Build history of the part. All positions in model axes, mm. A direction names the side the tool comes from. Give positions to 0.01 mm unless a question says otherwise; leave off trailing zeros. Write each loop counter-clockwise with the first axis right and the second up, starting at its lowest first coordinate (ties: lowest second). Pieces come first, ordered by that corner, then holes. Notation, with made-up numbers: (44, 49) -> (64, 49) arc R24 ccw to (64, 70) -> close; hole circle Ø8 at (13.5, -32). An arc over 180 degrees is marked (long way). Put each result on its own line as item: value.
from build123d import *

# Parameters (mm, degrees)
F2_DEPTH  = 12.5
F3_W      = 94
F3_H      = 30
F3_R      = 7.5
F4_DEPTH  = 18
F0_W      = 75
F0_H      = 20
F5_DEPTH  = 9.2
F6_W      = 30.81081
F6_H      = 70
F7_DEPTH  = 14
F8_W      = 35
F8_H      = 50.010137
F9_DEPTH  = 8.5
F10_W     = 60.514386
F10_H     = 9.2464
F11_DEPTH = 15


with BuildPart() as f2:
    # F1 (on Top) → F2 (new body)
    with BuildSketch(Plane.XY):
        Polygon((50.962807, 81.197856), (-43.037193, 81.197856), (-43.037193, 16.197856), (-43.037193, 11.091857), (-43.037193, -48.802144), (50.962807, -48.802144), align=None)
    extrude(amount=-F2_DEPTH)

    # F3 (on face) → F4 (join)
    with BuildSketch(Plane.XY):
        with Locations((3.962807, -33.802144)):
            Rectangle(F3_W, F3_H)
        with Locations((3.962807, -30.819066)):
            Circle(F3_R, mode=Mode.SUBTRACT)
    extrude(amount=F4_DEPTH)

    # F0 (on Top) → F5 (cut)
    with BuildSketch(Plane.XY):
        with Locations((4.462807, -28.802144)):
            Rectangle(F0_W, F0_H)
    extrude(amount=F5_DEPTH, mode=Mode.SUBTRACT)

    # F6 (on face) → F7 (join)
    with BuildSketch(Plane(origin=(0, 0, -12.5), x_dir=(1, 0, 0), z_dir=(0, 0, -1))):
        with Locations((5, -16.029622)):
            Rectangle(F6_W, F6_H)
        Polygon((10, -41.029622), (5, -41.029622), (0, -41.029622), (0, -22.373011), (10, -22.373011), align=None, mode=Mode.SUBTRACT)
        Polygon((0, 8.970378), (5, 8.970378), (10, 8.970378), (10, -11.889663), (0, -11.889663), align=None, mode=Mode.SUBTRACT)
    extrude(amount=F7_DEPTH)

    # F8 (on face) → F9 (cut)
    with BuildSketch(Plane(origin=(0, 0, -12.5), x_dir=(1, 0, 0), z_dir=(0, 0, -1))):
        with Locations((2.905405, -15.991903)):
            Rectangle(F8_W, F8_H)
    extrude(amount=F9_DEPTH, mode=Mode.SUBTRACT)

    # F10 (on face) → F11 (cut)
    with BuildSketch(Plane.XZ.offset(48.802144)):
        with Locations((-0.93579, 4.68071)):
            Rectangle(F10_W, F10_H)
    extrude(amount=-F11_DEPTH, mode=Mode.SUBTRACT)


solid = f2.part
1) Slice it at A-A (x = 24.5). Write the cut outline in (y, z), plus the area to 3 significant figures.
Filled sheet:
outline: (-48.8, -12.5) -> (81.2, -12.5) -> (81.2, 0) -> (-38.8, 0) -> (-38.8, 0.06) -> (-48.8, 0.06) -> close; (-48.8, 9.3) -> (-33.8, 9.3) -> (-33.8, 9.2) -> (-18.8, 9.2) -> (-18.8, 18) -> (-48.8, 18) -> close
area: 1,890 mm2
2) Slice it at B-B (y = 8). Write the cut outline in (x, z).
Filled sheet:
outline: (-43.04, -12.5) -> (50.96, -12.5) -> (50.96, 0) -> (-43.04, 0) -> close; (-10.41, -26.5) -> (0, -26.5) -> (0, -21) -> (-10.41, -21) -> close; (10, -26.5) -> (20.41, -26.5) -> (20.41, -21) -> (10, -21) -> close
3) Tool access for faces 5 (the cylindrical face through (2.986, -23.383, 13.538)), 6 (the flat face through (5, -8.97, -24)), 7 (the flat face through (5, -9.013, -17)), 8 (the flat face through (-10.405, 17, -23)): list every direction of +Z, -Z, +X, -X, +Y, -Y with a clear straight run to the whole face (end or side of a thin tool).
Filled sheet:
face 5: +Z
face 6: -Z
face 7: +X, -X
face 8: -Z, -X, +Y, -Y
4) Slice it at C-C (z = 6). Write the cut outline in (x, y).
Filled sheet:
outline: (-43.04, -48.8) -> (-31.19, -48.8) -> (-31.19, -38.8) -> (-33.04, -38.8) -> (-33.04, -18.8) -> (-43.04, -18.8) -> close; (29.32, -48.8) -> (50.96, -48.8) -> (50.96, -18.8) -> (41.96, -18.8) -> (41.96, -38.8) -> (29.32, -38.8) -> close
5) Wall check: L1, parallel to Z at x = -1.5, y = 19; L2, parallel to Z at x = -21, y = -40.5; L3, parallel to Z at x = 45.5, y = 27. Give the ranges that are in metal, low to high.
Filled sheet:
L1: -26.5 to -21, -12.5 to 0
L2: -12.5 to 0.06, 9.3 to 18
L3: -12.5 to 0
6) Pin check, flat tips, straight feed: pin 1 (9 mm diameter, centred on x = 4.5, y = 14.5, fed in from +Z); pin 2 (4.5 mm diameter, centred on x = 6, z = -23.5, fed in from +Y); pin 3 (6 mm diameter, centred on x = 6, z = -25, fed in from -Y); pin 4 (8 mm diameter, centred on y = 16.5, z = 1, fed in from +X). Stop position of each tip, or through.
Filled sheet:
pin 1: z = 0
pin 2: y = 51.03
pin 3: y = -18.97
pin 4: x = 50.96
7) Pull direction Y, two halves, no side cores. Call faces 1 (the flat face through (5, -18.97, -19)), 2 (the flat face through (3, 22, 0)), 3 (the flat face through (3, 17, -12.5)), 4 (the flat face through (5, 81.198, -6)): released by +Y, released by -Y, zero draft, split by the parting line, or undercut.
Filled sheet:
face 1: released by -Y
face 2: zero draft
face 3: undercut
face 4: released by +Y
8) Slice it at D-D (x = -6.5). Write the cut outline in (y, z).
Filled sheet:
outline: (-48.8, -12.5) -> (-18.97, -12.5) -> (-18.97, -26.5) -> (51.03, -26.5) -> (51.03, -12.5) -> (81.2, -12.5) -> (81.2, 0) -> (-38.8, 0) -> (-38.8, 0.06) -> (-48.8, 0.06) -> close; (-48.8, 9.3) -> (-33.8, 9.3) -> (-33.8, 9.2) -> (-18.8, 9.2) -> (-18.8, 18) -> (-48.8, 18) -> close; hole (-9.01, -21) -> (41, -21) -> (41, -12.5) -> (-9.01, -12.5) -> close
